```python
from build123d import *

# Parameters (mm, degrees)
BOX020_W          = 33
BOX020_H          = 70
BOX020_DEPTH      = 6
CYLINDER002_R     = 4.5
CYLINDER002_DEPTH = 4
BOX004_W          = 27
BOX004_H          = 4
BOX004_DEPTH      = 18
BOX005_W          = 4
BOX005_H          = 25
BOX005_DEPTH      = 18
BOX001_W          = 85
BOX001_H          = 60
BOX001_DEPTH      = 22
BOX008_W          = 8
BOX008_H          = 8
BOX008_DEPTH      = 10
BOX015_W          = 8
BOX015_H          = 5
BOX015_DEPTH      = 8
BOX016_W          = 8
BOX016_H          = 5
BOX016_DEPTH      = 8
CYLINDER_R        = 4
CYLINDER_DEPTH    = 84
BOX_W             = 90
BOX_H             = 70
BOX_DEPTH         = 27
CYLINDER005_R     = 5
CYLINDER005_DEPTH = 8
BOX009_W          = 3
BOX009_H          = 16
BOX009_DEPTH      = 3
CYLINDER004_R     = 8
CYLINDER004_DEPTH = 10


with BuildPart() as bottompedalhingecutout:
    # Box020 → Box020 (new body)
    with BuildSketch(Plane.XY.offset(21)):
        with Locations((16.5, 35)):
            Rectangle(BOX020_W, BOX020_H)
    extrude(amount=BOX020_DEPTH)


with BuildPart() as potentiometermountinghole:
    # Cylinder002 → Cylinder002 (new body)
    with BuildSketch(Plane(origin=(19.5, 39, 14), x_dir=(1, 0, 0), z_dir=(0, -1, 0))):
        Circle(CYLINDER002_R)
    extrude(amount=CYLINDER002_DEPTH)


with BuildPart() as potentiometerplate:
    # Box004 → Box004 (new body)
    with BuildSketch(Plane(origin=(6, 35, 5), x_dir=(1, 0, 0), z_dir=(0, 0, 1))):
        with Locations((13.5, 2)):
            Rectangle(BOX004_W, BOX004_H)
    extrude(amount=BOX004_DEPTH)


with BuildPart() as potentiometermount:
    # Box005 → Box005 (new body)
    with BuildSketch(Plane(origin=(2, 24.5, 5), x_dir=(1, 0, 0), z_dir=(0, 0, 1))):
        with Locations((2, 12.5)):
            Rectangle(BOX005_W, BOX005_H)
    extrude(amount=BOX005_DEPTH)

    # Fusion002: union PotentiometerPlate
    add(potentiometerplate.part)

    # Cut002: cut PotentiometerMountingHole
    add(potentiometermountinghole.part, mode=Mode.SUBTRACT)


with BuildPart() as bottompedalinsidebody:
    # Box001 → Box001 (new body)
    with BuildSketch(Plane(origin=(5, 5, 5), x_dir=(1, 0, 0), z_dir=(0, 0, 1))):
        with Locations((42.5, 30)):
            Rectangle(BOX001_W, BOX001_H)
    extrude(amount=BOX001_DEPTH)


with BuildPart() as wireholecutout:
    # Box008 → Box008 (new body)
    with BuildSketch(Plane(origin=(78, 62, 0), x_dir=(1, 0, 0), z_dir=(0, 0, 1))):
        with Locations((4, 4)):
            Rectangle(BOX008_W, BOX008_H)
    extrude(amount=BOX008_DEPTH)


with BuildPart() as obj1:
    # Box015 → Box015 (new body)
    with BuildSketch(Plane(origin=(61, 65, 7), x_dir=(1, 0, 0), z_dir=(0, 0, 1))):
        with Locations((4, 2.5)):
            Rectangle(BOX015_W, BOX015_H)
    extrude(amount=BOX015_DEPTH)


with BuildPart() as obj2:
    # Box016 → Box016 (new body)
    with BuildSketch(Plane(origin=(61, 0, 7), x_dir=(1, 0, 0), z_dir=(0, 0, 1))):
        with Locations((4, 2.5)):
            Rectangle(BOX016_W, BOX016_H)
    extrude(amount=BOX016_DEPTH)


with BuildPart() as bottompedalcutout:
    # Cylinder → Cylinder (new body)
    with BuildSketch(Plane(origin=(19.5, 77, 14), x_dir=(1, 0, 0), z_dir=(0, -1, 0))):
        Circle(CYLINDER_R)
    extrude(amount=CYLINDER_DEPTH)

    # Fusion: union BottomPedalInsideBody, WireHoleCutOut, obj1, obj2
    add(bottompedalinsidebody.part)
    add(wireholecutout.part)
    add(obj1.part)
    add(obj2.part)


with BuildPart() as pedalbodybottom:
    # Box → Box (new body)
    with BuildSketch(Plane.XY):
        with Locations((45, 35)):
            Rectangle(BOX_W, BOX_H)
    extrude(amount=BOX_DEPTH)

    # Cut: cut BottomPedalCutout
    add(bottompedalcutout.part, mode=Mode.SUBTRACT)


with BuildPart() as bottomspringholeinner:
    # Cylinder005 → Cylinder005 (new body)
    with BuildSketch(Plane(origin=(65, 35, 7), x_dir=(1, 0, 0), z_dir=(0, 0, 1))):
        Circle(CYLINDER005_R)
    extrude(amount=CYLINDER005_DEPTH)


with BuildPart() as bottomspringholecutout:
    # Box009 → Box009 (new body)
    with BuildSketch(Plane(origin=(63.5, 27, 8), x_dir=(1, 0, 0), z_dir=(0, 0, 1))):
        with Locations((1.5, 8)):
            Rectangle(BOX009_W, BOX009_H)
    extrude(amount=BOX009_DEPTH)

    # Fusion004: union BottomSpringHoleInner
    add(bottomspringholeinner.part)


with BuildPart() as bottompedal:
    # Cylinder004 → Cylinder004 (new body)
    with BuildSketch(Plane(origin=(65, 35, 5), x_dir=(1, 0, 0), z_dir=(0, 0, 1))):
        Circle(CYLINDER004_R)
    extrude(amount=CYLINDER004_DEPTH)

    # Cut004: cut BottomSpringHoleCutout
    add(bottomspringholecutout.part, mode=Mode.SUBTRACT)

    # Fusion007: union PotentiometerMount, PedalBodyBottom
    add(potentiometermount.part)
    add(pedalbodybottom.part)

    # Cut008: cut BottomPedalHingeCutout
    add(bottompedalhingecutout.part, mode=Mode.SUBTRACT)


solid = bottompedal.part
```
CAD build for the part. Positions are in the model's coordinates, mm. A direction names the side the tool comes from. Give positions to 0.01 mm unless a question says otherwise; leave off trailing zeros. Order: outer loops, then holes, each group sorted by start corner. A loop starts at its lowest first (then second) coordinate and runs counter-clockwise, first axis right, second up.
(1) Drill centre lines: L1, parallel to Y at x = 30, z = 7; L2, parallel to X at y = 66.95, z = 14; L3, parallel to Y at x = 78.5, z = 22.5. Where is each one in solid material? Low to high.
(2) Flat gauge pins, fed straight in: pin 1 (3 mm diameter, centred on x = 63.5, y = 35.5, fed in from +Z); pin 2 (1.5 mm diameter, centred on y = 3, z = 25, fed in from -X); pin 3 (4 mm diameter, centred on x = 80.5, y = 68, fed in from -Z). Where does each tip first touch, or does it go through?
(3) Saw through at C-C, the plane x = 19.5. Give the cut face in (y, z).
(4) Tool access for faces 1 (the flat face through (65, 29, 11)), 2 (the flat face through (82, 62, 2)), 3 (the flat face through (19, 35, 9)), 4 (the flat face through (69, 2, 11)), 5 (the flat face through (70.2, 35.1, 15)): list every direction of +Z, -Z, +X, -X, +Y, -Y with a clear straight run to the whole face (end or side of a thin tool).
(5) Saw through at A-A, the plane x = 65. State how many separate pieces and enclosed holes the cut face has, then the cut area to 3 significant figures.
(6) Saw through at D-D, the plane y = 51.5. Give the cut face in (x, z).
(7) Saw through at B-B, the plane z = 22.25. Give the cut face in (x, y), then the cut area to 3 significant figures.
(8) Mould opens along Y. For faces 6 (the flat face through (6, 44, 13)), 7 (the flat face through (78, 67, 5)), 8 (the flat face through (44, 70, 13)) say: released by +Y, released by -Y, zero draft, split by the parting line, or undercut.
Results found:
1. L1: y = 0 to 5, 35 to 39, 65 to 70
1. L2: x = 0 to 15.5, 23.5 to 61, 69 to 90
1. L3: y = 0 to 5, 65 to 70
2. pin 1: stops at z = 7
2. pin 2: stops at x = 33
2. pin 3: stops at z = 10
3. outline: (0, 0) - (70, 0) - (70, 10) - (65, 10) - (65, 5) - (39, 5) - (39, 9.5) - (35, 9.5) - (35, 5) - (5, 5) - (5, 10) - (0, 10) - close; (0, 18) - (5, 18) - (5, 21) - (0, 21) - close; (35, 18.5) - (39, 18.5) - (39, 21) - (35, 21) - close; (65, 18) - (70, 18) - (70, 21) - (65, 21) - close
4. face 1: +Y, -Y
4. face 2: +Z, -Z, +Y
4. face 3: +Z
4. face 4: -Y
4. face 5: +Z, +X
5. separate pieces: 5
5. enclosed holes: 0
5. area: 552 mm2
6. outline: (0, 0) - (90, 0) - (90, 5) - (5, 5) - (5, 21) - (0, 21) - close
7. outline: (33, 0) - (90, 0) - (90, 5) - (33, 5) - close; (33, 65) - (90, 65) - (90, 70) - (33, 70) - close
7. area: 570 mm2
8. face 6: undercut
8. face 7: zero draft
8. face 8: released by +Y
